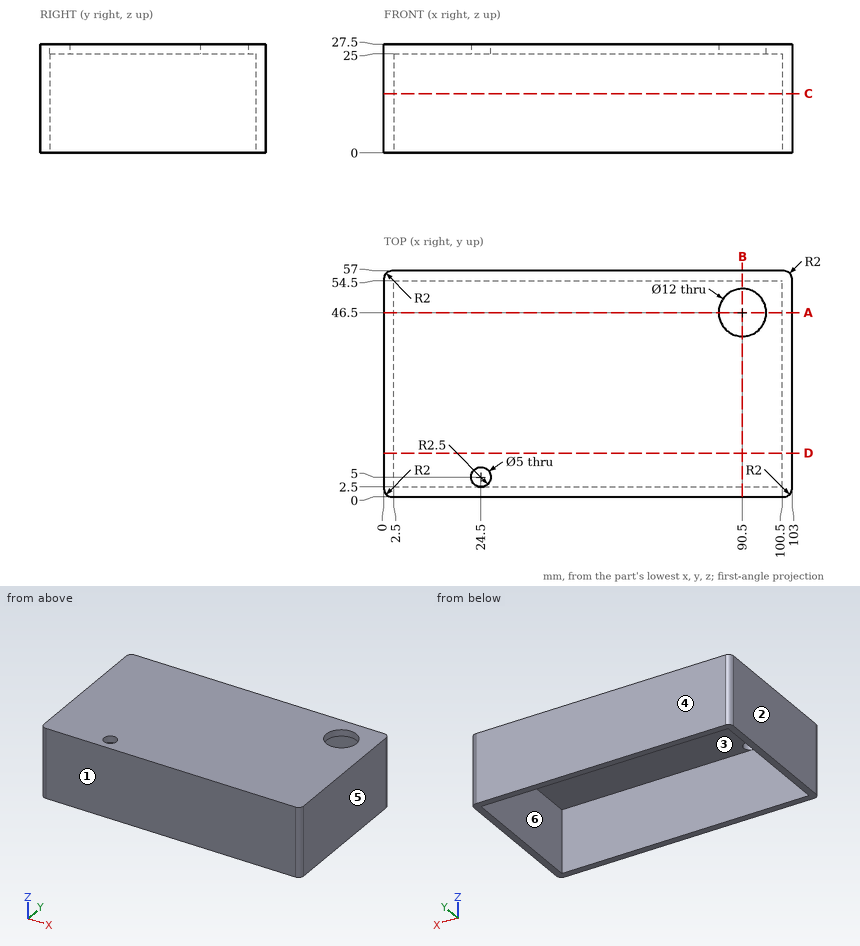
Geometry check sheet. Reference: drawing and pictorial views, mm from the part's lowest x, y, z. A direction names the side the tool comes from. Give positions to 0.01 mm unless a question says otherwise; leave off trailing zeros. Loops run counter-clockwise (first coordinate to the right, second up) from the corner with the lowest first, then second, coordinate; pieces in that order, holes last. Notation, with made-up numbers: M 5.25,-38.5 L 46.25,-38.5 A16 ccw 46.25,-31.5 Z; hole C -1.75,67 d7. An arc over 180 degrees is marked long. Use a Markdown table: item, result. Add a question column.
Q1. Mould release check, pull along Y, two halves, no side actions. Record for the marked faces 1, 2, 3 and 4: pulls with the +Y half, pulls with the -Y half, needs draft (parallel to the pull), parting line crosses it, or undercut.
Q2. Go/stop test with flat-tipped pins: pin 1 (8 mm diameter, centred on x = 27, y = 28.5, fed in from -Z); pin 2 (7 mm diameter, centred on x = 90.5, y = 46.5, fed in from +Z). Record where each tip stops, or that it passes through.
Q3. Sectioned sample at A-A, the plane y = 46.5. Record the cut outline in (x, z).
Q4. Tool access check on the marked faces 5 and 6. Record the directions out of +Z, -Z, +X, -X, +Y, -Y that give a thin tool (end or side, any length) a straight path to the whole face; none if there is none.
Q5. Sectioned sample at C-C, the plane z = 15. Record the cut outline in (x, y).
Q6. Scan lines: line 1 along Y through (x, z) = (85, 4.75); line 2 along X through (y, z) = (48, 5); line 3 along Y through (x, z) = (24.5, 26.6). Record each from-to range of solid material in increasing order. Write a range as [from, to].
Q7. Sectioned sample at B-B, the plane x = 90.5. Record the cut outline in (y, z), then the cut area to 4 significant figures.
Q8. Sectioned sample at D-D, the plane y = 11. Record the cut outline in (x, z), then the cut area to 4 significant figures.
Verdict:
| question | item | result |
|---|---|---|
| 1 | face 1 | pulls with the -Y half |
| 1 | face 2 | needs draft |
| 1 | face 3 | undercut |
| 1 | face 4 | pulls with the +Y half |
| 2 | pin 1 | z = 25 |
| 2 | pin 2 | through |
| 3 | outline | M 0,0 L 2.5,0 L 2.5,25 L 84.5,25 L 84.5,27.5 L 0,27.5 Z; M 96.5,25 L 100.5,25 L 100.5,0 L 103,0 L 103,27.5 L 96.5,27.5 Z |
| 4 | face 5 | +Z, -Z, +X, +Y, -Y |
| 4 | face 6 | -Z |
| 5 | outline | M 0,2 A2 ccw 2,0 L 101,0 A2 ccw 103,2 L 103,55 A2 ccw 101,57 L 2,57 A2 ccw 0,55 Z; hole M 2.5,2.5 L 100.5,2.5 L 100.5,54.5 L 2.5,54.5 Z |
| 6 | line 1 | [0, 2.5], [54.5, 57] |
| 6 | line 2 | [0, 2.5], [100.5, 103] |
| 6 | line 3 | [0, 2.5], [7.5, 57] |
| 7 | outline | M 0,0 L 2.5,0 L 2.5,25 L 40.5,25 L 40.5,27.5 L 0,27.5 Z; M 52.5,25 L 54.5,25 L 54.5,0 L 57,0 L 57,27.5 L 52.5,27.5 Z |
| 7 | area | 237.5 mm^2 |
| 8 | outline | M 0,0 L 2.5,0 L 2.5,25 L 100.5,25 L 100.5,0 L 103,0 L 103,27.5 L 0,27.5 Z |
| 8 | area | 382.5 mm^2 |
